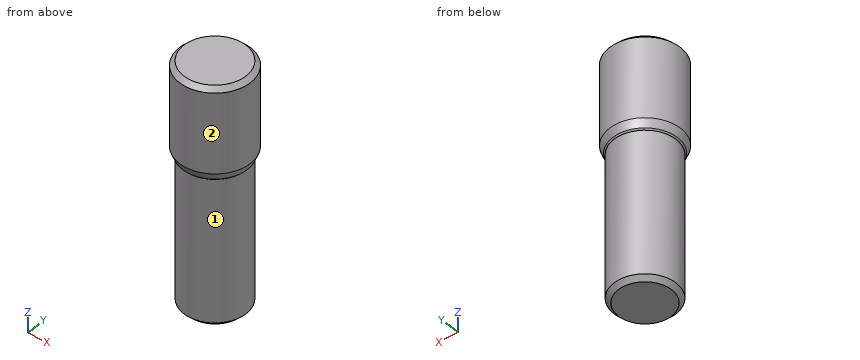
Autodesk Inventor part; units mm, degrees
ref_plane "YZ Plane" through (0, 0, 0) normal (1, 0, 0) x (0, 1, 0)
ref_plane "XZ Plane" through (0, 0, 0) normal (0, 1, 0) x (-1, 0, 0)
ref_plane "XY Plane" through (0, 0, 0) normal (0, 0, 1) x (1, 0, 0)
sketch "Sketch1" plane through (0, 0, 0) normal (0, 0, 1) x (1, 0, 0)
  circle A0 centre (0, 0) radius 3.5
  dimension "d0" = 7
extrude "Extrusion1" add sketch "Sketch1" along normal mid plane 17
sketch "Sketch2" plane through (0, 0, 8.5) normal (0, 0, 1) x (1, 0, 0)
  circle A0 centre (0, 0) radius 3.5
  circle A1 centre (0, 0) radius 4
  dimension "d3" = 8
extrude "Extrusion2" add sketch "Sketch2" along normal blind 10 contours A0 | A1
chamfer "Chamfer1" distance 0.5 angle 45 4 edges at (-3.5, 0, -8.5) (-3.5, 0, 8.5) (-4, 0, 8.5) (-4, 0, 18.5)
properties part number "as gearbox" material "Stainless Steel"
The listing builds one solid part. Answer for the finished solid, in the listing's coordinates (mm). Face numbers are marked on the shaded views. A direction names the side the tool comes from. Give positions to 0.01 mm unless a question says otherwise; leave off trailing zeros. Loops run counter-clockwise (first coordinate to the right, second up) from the corner with the lowest first, then second, coordinate; pieces in that order, holes last. Notation, with made-up numbers: (-36, 80.25) - (-8, 80.25) arc R26 cw to (-8, 108.25) - close; hole circle Ø4 at (54.25, 86). An arc over 180 degrees is marked (long way). Write each question's results on one line, items separated by ' | '.
1. Find section D-D, the plane z = 14.75. Write down the section's boundary in (x, y).
Resolved:
outline: circle Ø8 at (0, 0)
2. Find section A-A, the plane y = 0. Write down the section's boundary in (x, z).
Resolved:
outline: (-4, 9) - (-3.65, 8.15) - (-3.5, 8) - (-3.5, -8) - (-3, -8.5) - (3, -8.5) - (3.5, -8) - (3.5, 8) - (3.65, 8.15) - (4, 9) - (4, 18) - (3.5, 18.5) - (-3.5, 18.5) - (-4, 18) - close
3. Flat-ended cylindrical pins translate along their axes: P1, Ø3, axis at y = -2, z = 12.5, coming from the -X side; P2, Ø3, axis at x = 0.5, z = 7, coming from the -Y side; P3, Ø2, axis at y = -0.5, z = 3, coming from the -X side; P4, Ø3, axis at x = -1.5, z = 12.5, coming from the -Y side. Find the tip coordinate at first contact, or state that the pin passes through.
Resolved:
P1: stops at x = -3.97 | P2: stops at y = -3.78 | P3: stops at x = -3.5 | P4: stops at y = -4
4. Find section C-C, the plane z = 0.5. Write down the section's boundary in (x, y), then the cut area to 3 significant figures.
Resolved:
outline: circle Ø7 at (0, 0) | area: 38.5 mm^2
5. Which of the six approach directions +Z, -Z, +X, -X, +Y, -Y give full straight-line access (tool end or side, diameter ignored) to the marked faces 1 and 2?
Resolved:
face 1: -Z | face 2: +Z, -Z
6. Consider probe 1 along Y at (x, z) = (0, 7); probe 2 along Y at (x, z) = (2.25, -7.25); probe 3 along X at (y, z) = (1.75, 5). Determine where each line is inside the solid, lowest interval first. Write a range as from..to.
Resolved:
probe 1: y = -3.5..3.5 | probe 2: y = -2.68..2.68 | probe 3: x = -3.03..3.03
